Design review of the part shown in the three views and the two pictorial views. Dimensions are in mm from the part's minimum x, y and z. A direction names the side the tool comes from. Give positions to 0.01 mm unless a question says otherwise; leave off trailing zeros. Order: outer loops, then holes, each group sorted by start corner. A loop starts at its lowest first (then second) coordinate and runs counter-clockwise, first axis right, second up.
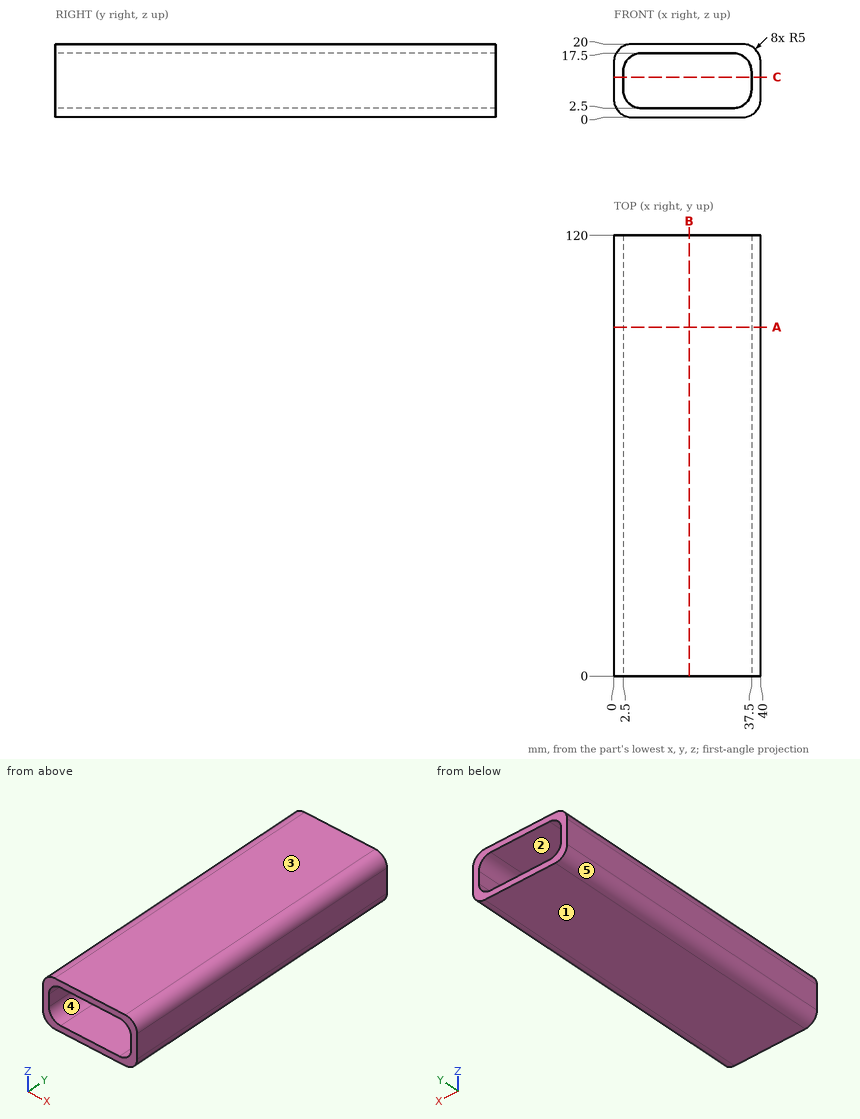
Item 1: Take a section at C-C (z = 11). Give the boundary of the cut face in (x, y).
Values found:
outline: (0, 0) - (2.5, 0) - (2.5, 120) - (0, 120) - close; (37.5, 0) - (40, 0) - (40, 120) - (37.5, 120) - close
Item 2: For the marked faces 1 and 2, list the 3-axis set-ups (+Z, -Z, +X, -X, +Y, -Y) from which the entire face can be reached by the end or side of a thin tool; tool diameter is ignored.
Values found:
face 1: -Z, +X, -X, +Y, -Y
face 2: +Y, -Y
Item 3: Take a section at A-A (y = 95). Give the boundary of the cut face in (x, z).
Values found:
outline: (0, 5) arc R5 ccw to (5, 0) - (35, 0) arc R5 ccw to (40, 5) - (40, 15) arc R5 ccw to (35, 20) - (5, 20) arc R5 ccw to (0, 15) - close; hole (2.5, 7.5) arc R5 ccw to (7.5, 2.5) - (32.5, 2.5) arc R5 ccw to (37.5, 7.5) - (37.5, 12.5) arc R5 ccw to (32.5, 17.5) - (7.5, 17.5) arc R5 ccw to (2.5, 12.5) - close
Item 4: For line 1 (X direction, y = 86.5, z = 11.5); line 2 (Z direction, x = 25.5, y = 52); line 3 (X direction, y = 12, z = 5.25), list the stretches that pass through material, from the lowest coordinate up.
Values found:
line 1: x = 0 to 2.5, 37.5 to 40
line 2: z = 0 to 2.5, 17.5 to 20
line 3: x = 0 to 3.03, 36.97 to 40
Item 5: Draft analysis for pull direction Z (two halves, no side actions). For the marked faces 3, 4 and 5, state which applies: released by +Z, released by -Z, zero draft, split by the parting line, or undercut.
Values found:
face 3: released by +Z
face 4: undercut
face 5: released by -Z
Item 6: Take a section at B-B (x = 20.5). Give the boundary of the cut face in (y, z).
Values found:
outline: (0, 0) - (120, 0) - (120, 2.5) - (0, 2.5) - close; (0, 17.5) - (120, 17.5) - (120, 20) - (0, 20) - close
